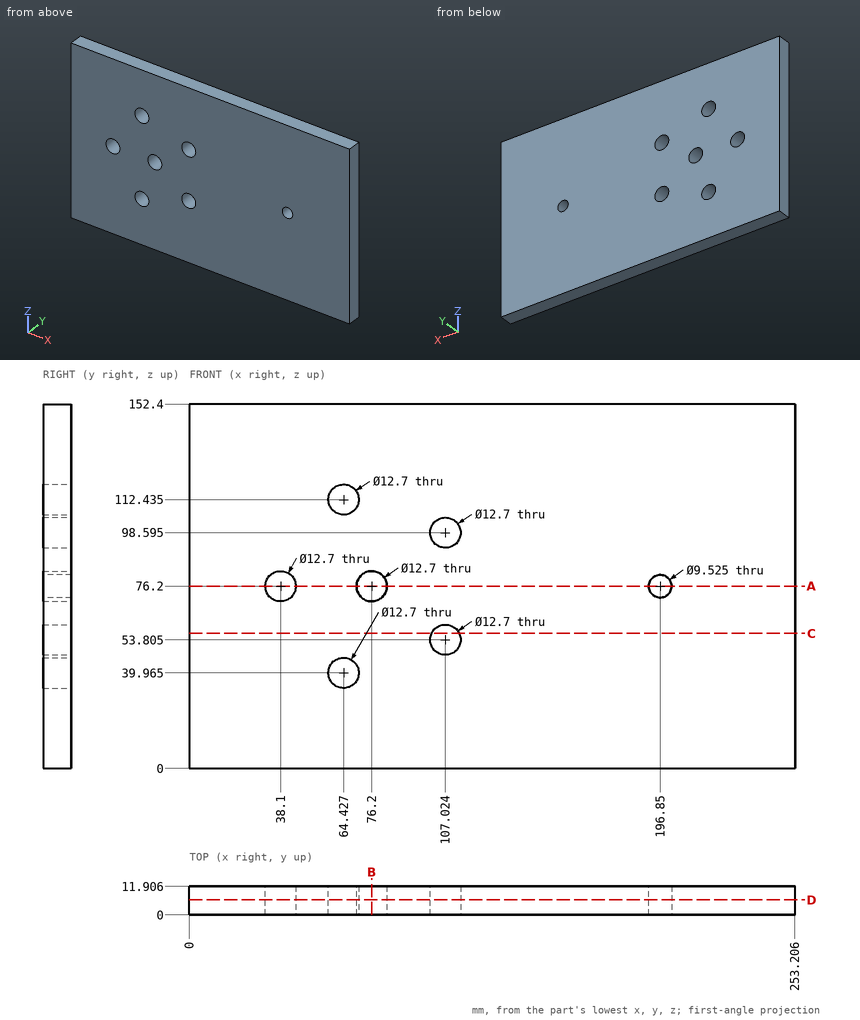
Can you work these out from the drawing? Everything is in mm from the part's minimum corner. Give positions to 0.01 mm unless a question says otherwise; leave off trailing zeros. Order: outer loops, then holes, each group sorted by start corner. A loop starts at its lowest first (then second) coordinate and runs counter-clockwise, first axis right, second up. Notation, with made-up numbers: M -15,-20 L 17,-20 A23 ccw 17,13 Z; hole C 16,-20.5 d4. An arc over 180 degrees is marked long. One line per item, written item: value.
Item 1: If we section it at C-C on z = 56.5: Write out the boundary of the cut face in (x, y).
Verdict:
outline: M 0,0 L 101.27,0 L 101.27,11.91 L 0,11.91 Z; M 112.77,0 L 253.21,0 L 253.21,11.91 L 112.77,11.91 Z
Item 2: If we section it at D-D on y = 6.25: State how many separate pieces and enclosed holes the cut face has, and give its area (3 significant figures).
Verdict:
separate pieces: 1
enclosed holes: 7
area: 37,800 mm2
Item 3: For pin 1 (10 mm diameter, centred on x = 107.02, z = 53.81, fed in from +Y); pin 2 (4 mm diameter, centred on x = 75, y = 5.5, fed in from -Z), each with a flat end and sliding along its axis, tell me the tip position at first contact or that it passes through.
Verdict:
pin 1: through
pin 2: z = 0
Item 4: If we section it at B-B on x = 76.2: Write out the boundary of the cut face in (y, z).
Verdict:
outline: M 0,0 L 11.91,0 L 11.91,69.85 L 0,69.85 Z; M 0,82.55 L 11.91,82.55 L 11.91,152.4 L 0,152.4 Z
Item 5: If we section it at A-A on z = 76.2: Write out the boundary of the cut face in (x, y).
Verdict:
outline: M 0,0 L 31.75,0 L 31.75,11.91 L 0,11.91 Z; M 44.45,0 L 69.85,0 L 69.85,11.91 L 44.45,11.91 Z; M 82.55,0 L 192.09,0 L 192.09,11.91 L 82.55,11.91 Z; M 201.61,0 L 253.21,0 L 253.21,11.91 L 201.61,11.91 Z
Item 6: Please list where these lines run through material, in increasing order: line 1 (X direction, y = 7.5, z = 76.2); line 2 (Z direction, x = 196.85, y = 8); line 3 (Z direction, x = 76.2, y = 4).
Verdict:
line 1: 0 to 31.75, 44.45 to 69.85, 82.55 to 192.09, 201.61 to 253.21
line 2: 0 to 71.44, 80.96 to 152.4
line 3: 0 to 69.85, 82.55 to 152.4
